```python
from build123d import *

# Parameters (mm, degrees)
PAD001_DEPTH        = 2
PAD002_DEPTH        = 3.5
PAD003_DEPTH        = 1.25
CYLINDER_R          = 1
CYLINDER_DEPTH      = 20
LINEARPATTERN_COUNT = 3
LINEARPATTERN_PITCH = 3
POCKET008_DEPTH     = 0.4


with BuildPart() as part:
    # Sketch008 → Pad001 (new body)
    with BuildSketch(Plane.XZ):
        with BuildLine():
            ThreePointArc((-6.25, 3.75), (-10, 0), (-6.25, -3.75))
            Line((-6.25, -3.75), (6.25, -3.75))
            ThreePointArc((6.25, -3.75), (10, 0), (6.25, 3.75))
            Line((6.25, 3.75), (-6.25, 3.75))
        make_face()
    extrude(amount=PAD001_DEPTH)

    # Sketch010 → Pad002 (join)
    with BuildSketch(Plane.XZ):
        with BuildLine():
            ThreePointArc((-11.25, 5.75), (-17, 0), (-11.25, -5.75))
            Line((-11.25, -5.75), (11.25, -5.75))
            ThreePointArc((11.25, -5.75), (17, 0), (11.25, 5.75))
            Line((11.25, 5.75), (-11.25, 5.75))
        make_face()
    extrude(amount=-PAD002_DEPTH)

    # Sketch011 → Pad003 (join)
    with BuildSketch(Plane.XY.offset(4.5)):
        Polygon((-7, 0), (-7, 13), (-4, 13), (-4, 9), (-2, 9), (-2, 13), (1, 13), (1, 0), align=None)
    extrude(amount=PAD003_DEPTH)

    # Cylinder → Cylinder (cut)
    with BuildSketch(Plane(origin=(-3, -2, -10), x_dir=(1, 0, 0), z_dir=(0, 0, 1))):
        Circle(CYLINDER_R)
    cylinder = extrude(amount=CYLINDER_DEPTH, mode=Mode.SUBTRACT)

    # LinearPattern: Cylinder ×3
    with Locations(*[(i * LINEARPATTERN_PITCH, 0, 0) for i in range(1, LINEARPATTERN_COUNT)]):
        add(cylinder, mode=Mode.SUBTRACT)

    # Sketch012 → Pocket008 (cut)
    with BuildSketch(Plane.XZ.offset(2)):
        with BuildLine():
            ThreePointArc((-4.5, 0), (-6.5, 2), (-8.5, 0))
            Line((-8.5, 0), (-8.5, -1.6))
            Line((-8.5, -1.6), (-4.5, -1.6))
            Line((-4.5, -1.6), (-4.5, 0))
        make_face()
        with BuildLine():
            ThreePointArc((-5.1, 0), (-6.5, 1.4), (-7.9, 0))
            Line((-7.9, -1), (-7.9, 0))
            Line((-5.1, -1), (-7.9, -1))
            Line((-5.1, 0), (-5.1, -1))
        make_face(mode=Mode.SUBTRACT)
        with BuildLine():
            ThreePointArc((5.520204, 1), (6.5, -1.4), (7.479796, 1))
            Line((7.479796, 1), (7.899708, 1.428571))
            ThreePointArc((5.100292, 1.428571), (6.5, -2), (7.899708, 1.428571))
            Line((5.520204, 1), (5.100292, 1.428571))
        make_face()
    extrude(amount=-POCKET008_DEPTH, mode=Mode.SUBTRACT)


solid = part.part
```
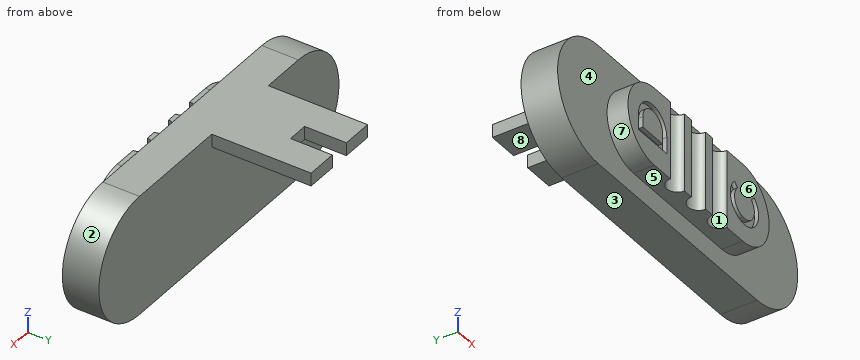
The listing builds one solid part. Answer for the finished solid, in the listing's coordinates (mm). Face numbers are marked on the shaded views. A direction names the side the tool comes from. Coordinates: 2 decimals unless noted, no trailing zeros. Write each loop counter-clockwise with the first axis right and the second up, starting at its lowest first coordinate (ties: lowest second). Pieces come first, ordered by that corner, then holes. Notation, with made-up numbers: (23.25, 45.25) - (65.25, 45.25) arc R24 ccw to (65.25, 65.25) - close; hole circle Ø1 at (3, 7). An arc over 180 degrees is marked (long way). Return JSON: item names as keys, results as strings. Group by question number.
1. Which of the six approach directions +Z, -Z, +X, -X, +Y, -Y give full straight-line access (tool end or side, diameter ignored) to the marked faces 4, 5, 6, 7 and 8?
2. A cutting plane is placed at B-B, the plane z = 2.75. Determine the outline of the cut face in (x, y), plus the area to 3 significant figures.
3. Determine the mould class of the marked faces 1, 2 and 3 for opening direction X: released by +X, released by -X, zero draft, split by the parting line, or undercut.
4. Straight lines are drawn through the part: L1, parallel to Z at x = 6.5, y = -1.8; L2, parallel to Z at x = 6.5, y = -0.25; L3, parallel to Y at x = -5.5, z = 0.5. For each, find the intervals that lie inside material, in ascending order.
5. Given pin 1 (1 mm diameter, centred on y = 10, z = 5, fed in from +X); pin 2 (2.5 mm diameter, centred on x = -2.5, y = 8.5, fed in from -Z); pin 3 (3.5 mm diameter, centred on x = -3.5, z = -1, fed in from +Y); pin 4 (1 mm diameter, centred on x = 3, y = 8, fed in from +Z), each flat-ended and moving along its own axis, determine where each tip first touches the part or whether it passes through.
6. A cutting plane is placed at A-A, the plane x = 3. Determine the outline of the cut face in (y, z), plus the area to 4 significant figures.
7. A cutting plane is placed at C-C, the plane y = 5.5. Determine the outline of the cut face in (x, z), plus the area to 3 significant figures.
8. A cutting plane is placed at D-D, the plane x = -3. Determine the outline of the cut face in (y, z).
Ans:
{
 "1": {"face 4": "-Y", "face 5": "-Z, +X, -X, -Y", "face 6": "+Z, -Z, +X, -X, -Y", "face 7": "-X, -Y", "face 8": "-Z, +X, -X, +Y"},
 "2": {"outline": "(-16.3, 0) - (-8.8, 0) - (-8.8, -2) - (-4, -2) arc R1 cw to (-2, -2) - (-1, -2) arc R1 cw to (1, -2) - (2, -2) arc R1 cw to (4, -2) - (8.8, -2) - (8.8, 0) - (16.3, 0) - (16.3, 3.5) - (-16.3, 3.5) - close", "area": "145 mm²"},
 "3": {"face 1": "undercut", "face 2": "released by +X", "face 3": "zero draft"},
 "4": {"L1": "-3.74 to -2, -1.4 to 3.74", "L2": "-3.74 to 3.74", "L3": "-2 to 3.5"},
 "5": {"pin 1": "x = 1", "pin 2": "z = 4.5", "pin 3": "y = 3.5", "pin 4": "through"},
 "6": {"outline": "(-1, -3.75) - (0, -3.75) - (0, -5.75) - (3.5, -5.75) - (3.5, 5.75) - (0, 5.75) - (0, 3.75) - (-1, 3.75) - close", "area": "47.75 mm²"},
 "7": {"outline": "(-7, 4.5) - (1, 4.5) - (1, 5.75) - (-7, 5.75) - close", "area": "10.0 mm²"},
 "8": {"outline": "(-1, -3.75) - (0, -3.75) - (0, -5.75) - (3.5, -5.75) - (3.5, 4.5) - (9, 4.5) - (9, 5.75) - (0, 5.75) - (0, 3.75) - (-1, 3.75) - close"}
}
